```python
from build123d import *


with BuildPart() as part:
    # Inlet Fairlead Liner Profile → Inlet Fairlead Liner Feature (revolve)
    with BuildSketch(Plane(origin=(3.258206564, -5.512003586, 12.159792439), x_dir=(0.9714880974430896, 0.09788446030256422, -0.21593866943574938), z_dir=(0.23708833064156934, -0.4010892811605493, 0.8848256958360261)), mode=Mode.PRIVATE) as inlet_fairlead_liner_feature_sk:
        with BuildLine():
            Line((-23.152018399, -30.892753147), (-23.579443274, -34.869851081))
            Line((-23.579443274, -34.869851081), (-22.634882515, -34.971364489))
            Line((-22.634882515, -34.971364489), (-23.062307391, -38.948462423))
            add(Edge.make_bspline(
                [(-23.062307391, -38.948462423), (-23.13354487, -39.611312079), (-24.199056833, -40.167305516), (-24.270294312, -40.830155171)],
                knots=[0, 0, 0, 0, 1, 1, 1, 1], degree=3))
            ThreePointArc((-24.270294312, -40.830155171), (-26.470944377, -44.860719778), (-30.877078526, -46.154664759))
            Line((-30.877078526, -46.154664759), (-31.871353009, -46.04780854))
            Line((-31.871353009, -46.04780854), (-25.165141347, -40.733984574))
            Line((-25.165141347, -40.733984574), (-24.951428909, -38.745435607))
            Line((-24.951428909, -38.745435607), (-25.945703393, -38.638579389))
            Line((-25.945703393, -38.638579389), (-25.731990955, -36.650030422))
            Line((-25.731990955, -36.650030422), (-24.737716471, -36.75688664))
            Line((-24.737716471, -36.75688664), (-24.096579158, -30.79123974))
            Line((-24.096579158, -30.79123974), (-23.152018399, -30.892753147))
        make_face()
    revolve(inlet_fairlead_liner_feature_sk.sketch.rotate(Axis((-17.253555798, -35.915165888, 3.874224953), (-0.10380954475082989, -0.9160389667138149, -0.38742249532069234)), 283.790724011), axis=Axis((-17.253555798, -35.915165888, 3.874224953), (-0.10380954475082989, -0.9160389667138149, -0.38742249532069234)))


with BuildPart() as body_2:
    # Mirror1: mirrored copy
    add(part.part.mirror(Plane(origin=(0, 0, 0), x_dir=(0, 0, 1), z_dir=(0, -1, 0))))


solid = body_2.part
```
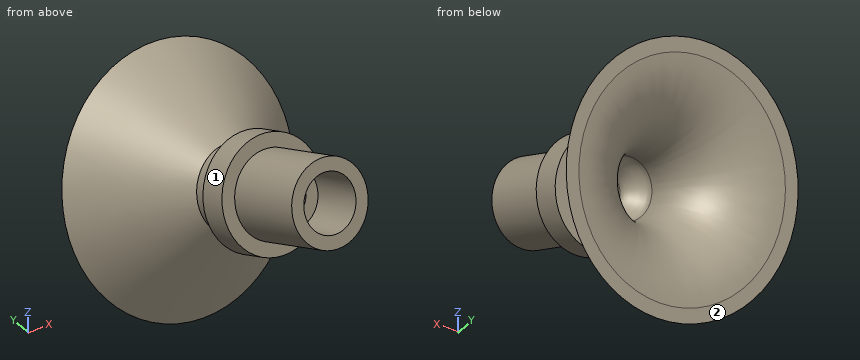
Here's how the part is built. I have some questions about the finished solid (model axes, mm). Face numbers are marked on the shaded views. Round coordinates to 2 decimals unless told otherwise and drop trailing zeros. Answer in a Markdown table with one row per item.
Item 1: If I drill on L1, parallel to Y at x = -15.25, z = -0.5; L2, parallel to Y at x = -16.5, z = 5; L3, parallel to X at y = 49, z = -0.25, over which ranges is the centre line in solid material (lowest first)? Write a range as from..to.
A:
| item | result |
|---|---|
| L1 | y = 40.84..43.03, 45.31..49.71 |
| L2 | y = 37.98..40.39, 52.66..53.94 |
| L3 | x = -26.2..-22.18, -15.76..-12.63 |
Item 2: I'm going to push flat-ended pins straight in: pin 1 (4 mm diameter, centred on x = -15, z = 2.5, fed in from -Y); pin 2 (4 mm diameter, centred on x = -18, y = 37, fed in from -Z); pin 3 (1 mm diameter, centred on x = -18, z = -6, fed in from -Y); pin 4 (5 mm diameter, centred on x = -17.5, y = 39, fed in from +Z). Where does each tip first touch, or does it pass through?
A:
| item | result |
|---|---|
| pin 1 | stops at y = 34.86 |
| pin 2 | stops at z = -0.68 |
| pin 3 | stops at y = 45.03 |
| pin 4 | stops at z = 6.64 |
Item 3: Thinking about a two-plate mould opening in Y: for the marked faces 1 and 2, which applies, +Y half, -Y half, draft (parallel to the pull), parting line (faces both ways), or undercut?
A:
| item | result |
|---|---|
| face 1 | undercut |
| face 2 | +Y half |
Item 4: Imagine slicing it at A-A, the plane x = -14.75. State how many separate pieces and enclosed holes the cut face has, and give its area (3 significant figures).
A:
| item | result |
|---|---|
| separate pieces | 3 |
| enclosed holes | 0 |
| area | 62.2 mm2 |
